```python
from build123d import *
from OCP.BRepFilletAPI import BRepFilletAPI_MakeFillet

# Parameters (mm, degrees)
EXTRUDE_1_DEPTH           = 7.6
SKETCH_3_R                = 1.65
CUT_EXTRUDE_2_DEPTH       = 25.678475018
SKETCH_5_W                = 30
SKETCH_5_H                = 14
EXTRUDE_3_DEPTH           = 3
CUT_EXTRUDE_7_DEPTH       = 0.2
EXTRUDE_9_DEPTH           = 4.5
EXTRUDE_9_DEPTH_BACK      = 1.5
SKETCH_24_R               = 2
CUT_EXTRUDE_8_DEPTH       = 52.317437946
EXTRUDE_10_DEPTH          = 4.5
EXTRUDE_10_DEPTH_BACK     = 1.5
SKETCH_28_R               = 2
CUT_EXTRUDE_9_DEPTH       = 10
FILLET_1_R                = 5
EXTRUDE_11_DEPTH          = 4.5
FILLET_3_R                = 2.2
EXTRUDE_12_DEPTH          = 1.5
SKETCH_33_R               = 4.1
CUT_EXTRUDE_10_DEPTH      = 4.2
CUT_EXTRUDE_START         = -4.2
SKETCH_35_R               = 4.1
CUT_EXTRUDE_11_DEPTH      = 4.2
SKETCH_36_W               = 21
SKETCH_36_H               = 3.5
CUT_EXTRUDE_12_DEPTH      = 30
EXTRUDE_16_DEPTH          = 16
SKETCH_44_R               = 1.6
CUT_EXTRUDE_15_DEPTH      = 6
FILLET_4_R1               = 2
FILLET_4_R2               = 1
FILLET_5_R                = 2
FILLET_4_OF_MIRROR_1_R1   = 2
FILLET_4_OF_MIRROR_1_R2   = 1
FILLET_5_OF_MIRROR_1_R    = 2
MIRROR_START              = -11
MIRROR_2_DEPTH            = 6
MIRROR_2_2_OUTLINE_R      = 1.6
MIRROR_2_2_DEPTH          = 3
SKETCH_45_W               = 21
SKETCH_45_H               = 2
CUT_EXTRUDE_16_DEPTH      = 85.096611109
CUT_EXTRUDE_17_DEPTH      = 87.210440203
CUT_EXTRUDE_17_DEPTH_BACK = 87.210440203
FILLET_6_R                = 0.5


# Read off the part's stored shape, not the designer's step: 镜向2
with BuildPart() as part:
    # 草图1 → 凸台-拉伸1 (new body)
    with BuildSketch(Plane(origin=(0, 0, 0), x_dir=(1, 0, 0), z_dir=(0, 1, 0))):
        with BuildLine():
            Line((0, 5), (15, 5))
            Line((15, 5), (22.940512837, 5))
            Line((22.940512837, 5), (20, 0))
            ThreePointArc((20, 0), (18.535533906, -3.535533906), (15, -5))
            Line((15, -5), (0, -5))
            ThreePointArc((0, -5), (-3.535533906, -3.535533906), (-5, 0))
            Line((-5, 0), (-7.940512837, 5))
            Line((-7.940512837, 5), (0, 5))
        make_face()
    extrude(amount=EXTRUDE_1_DEPTH)

    # 草图3 → 切除-拉伸2 (cut, through all)
    with BuildSketch(Plane(origin=(0, 7.6, 0), x_dir=(1, 0, 0), z_dir=(0, 1, 0))):
        with Locations(Location((0, 0, 0), (0, 0, 270))):
            Circle(SKETCH_3_R)
        with Locations(Location((15, 0, 0), (0, 0, 270))):
            Circle(SKETCH_3_R)
    extrude(amount=-CUT_EXTRUDE_2_DEPTH, mode=Mode.SUBTRACT)

    # 草图5 → 凸台-拉伸3 (add)
    with BuildSketch(Plane(origin=(0, 0, -5), x_dir=(-1, 0, 0), z_dir=(0, 0, -1))):
        with Locations((-7.5, 3.8)):
            Rectangle(SKETCH_5_W, SKETCH_5_H)
    extrude(amount=EXTRUDE_3_DEPTH)

    # 草图10 → 切除-拉伸7 (cut)
    with BuildSketch(Plane.XZ):
        with BuildLine():
            Line((0, 5), (15, 5))
            ThreePointArc((15, 5), (20, 0), (15, -5))
            Line((15, -5), (0, -5))
            ThreePointArc((0, -5), (-5, 0), (0, 5))
        make_face()
    extrude(amount=-CUT_EXTRUDE_7_DEPTH, mode=Mode.SUBTRACT)

    # 草图21 → 凸台-拉伸9 (add, two sides: drawn at the far end of the back side and taken through both)
    with BuildSketch(Plane(origin=(22.5, 0, 0), x_dir=(0, 0, -1), z_dir=(1, 0, 0)).offset(-EXTRUDE_9_DEPTH_BACK)):
        with BuildLine():
            Line((5, 10.8), (29, 10.8))
            ThreePointArc((29, 10.8), (36, 3.8), (29, -3.2))
            Line((29, -3.2), (5, -3.2))
            Line((5, -3.2), (5, 10.8))
        make_face()
    extrude(amount=EXTRUDE_9_DEPTH + EXTRUDE_9_DEPTH_BACK)

    # 草图24 → 切除-拉伸8 (cut, through all)
    with BuildSketch(Plane(origin=(27, 0, 0), x_dir=(0, 0, -1), z_dir=(1, 0, 0))):
        with Locations((28, 4.5)):
            Circle(SKETCH_24_R)
    extrude(amount=-CUT_EXTRUDE_8_DEPTH, mode=Mode.SUBTRACT)

    # 草图25 → 凸台-拉伸10 (add, two sides: drawn at the far end of the back side and taken through both)
    with BuildSketch(Plane.ZY.offset(7.5).offset(-EXTRUDE_10_DEPTH_BACK)):
        with BuildLine():
            Line((-5, -3.2), (-29, -3.2))
            ThreePointArc((-29, -3.2), (-36, 3.8), (-29, 10.8))
            Line((-29, 10.8), (-5, 10.8))
            Line((-5, 10.8), (-5, -3.2))
        make_face()
    extrude(amount=EXTRUDE_10_DEPTH + EXTRUDE_10_DEPTH_BACK)

    # 草图28 → 切除-拉伸9 (cut)
    with BuildSketch(Plane(origin=(-6, 0, 0), x_dir=(0, 0, -1), z_dir=(1, 0, 0))):
        with Locations((28, 4.5)):
            Circle(SKETCH_28_R)
    extrude(amount=-CUT_EXTRUDE_9_DEPTH, mode=Mode.SUBTRACT)

    # 圆角1
    fillet_1_edges = [part.edges().sort_by_distance(p)[0] for p in [
        (-6, 3.8, -8),
        (21, 3.8, -8),
    ]]
    fillet(fillet_1_edges, radius=FILLET_1_R)

    # 草图30 → 凸台-拉伸11 (add)
    with BuildSketch(Plane(origin=(0, 7.6, 0), x_dir=(1, 0, 0), z_dir=(0, 1, 0))):
        Polygon((10, -70), (13.5, -70), (13.5, -75), (1.5, -75), (1.5, -70), (5, -70), (5, 2.116473595), (10, 2.116473595), align=None)
    extrude(amount=EXTRUDE_11_DEPTH)

    # 圆角3
    fillet_3_edges = [part.edges().sort_by_distance(p)[0] for p in [
        (-12, 3.8, -5),
        (-7.940512837, 3.8, -5),
        (22.940512837, 3.8, -5),
        (27, 3.8, -5),
    ]]
    fillet(fillet_3_edges, radius=FILLET_3_R)

    # 草图31 → 凸台-拉伸12 (add)
    with BuildSketch(Plane.XZ.offset(-7.6)):
        Polygon((5, 70), (5, 5), (10, 5), (10, 70), (13.5, 70), (13.5, 75), (1.5, 75), (1.5, 70), align=None)
    extrude(amount=EXTRUDE_12_DEPTH)

    # 草图33 → 切除-拉伸10 (cut)
    with BuildSketch(Plane.ZY.offset(-21)):
        with Locations((-28, 4.5)):
            Circle(SKETCH_33_R)
    extrude(amount=-CUT_EXTRUDE_10_DEPTH, mode=Mode.SUBTRACT)

    # 草图35 → 切除-拉伸11 (cut)
    with BuildSketch(Plane(origin=(-6, 0, 0), x_dir=(0, 0, -1), z_dir=(1, 0, 0)).offset(CUT_EXTRUDE_START)):
        with Locations(Location((28, 4.5, 0), (0, 0, 180))):
            Circle(SKETCH_35_R)
    extrude(amount=CUT_EXTRUDE_11_DEPTH, mode=Mode.SUBTRACT)

    # 草图36 → 切除-拉伸12 (cut)
    with BuildSketch(Plane(origin=(0, 10.8, 0), x_dir=(1, 0, 0), z_dir=(0, 1, 0))):
        with Locations((7.5, 6.75)):
            Rectangle(SKETCH_36_W, SKETCH_36_H)
    extrude(amount=-CUT_EXTRUDE_12_DEPTH, mode=Mode.SUBTRACT)

    # 草图41 → 凸台-拉伸16 (add)
    with BuildSketch(Plane(origin=(0, 10.8, 0), x_dir=(1, 0, 0), z_dir=(0, 1, 0))):
        Polygon((17.5, 11), (11.5, 11), (11.5, 8), (18, 8), (18, 5), (24.8, 5), (24.8, 11), align=None)
    extrude_16 = extrude(amount=EXTRUDE_16_DEPTH)

    # 草图44 → 切除-拉伸15 (cut)
    with BuildSketch(Plane(origin=(0, 0, -11), x_dir=(-1, 0, 0), z_dir=(0, 0, -1))):
        with Locations((-14.5, 23.3)):
            Circle(SKETCH_44_R)
    cut_extrude_15 = extrude(amount=-CUT_EXTRUDE_15_DEPTH, mode=Mode.SUBTRACT)

    # 圆角4: one fillet with a radius per group of edges: ONE call of the kernel's fillet builder (fillet() takes one radius for all edges)
    fillet_4_edges_1 = [part.edges().sort_by_distance(p)[0] for p in [
        (11.5, 10.8, -9.5),
    ]]
    fillet_4_edges_2 = [part.edges().sort_by_distance(p)[0] for p in [
        (11.5, 26.8, -9.5),
    ]]
    fillet_4 = BRepFilletAPI_MakeFillet(part.part.solid().wrapped)
    for e in fillet_4_edges_1:
        fillet_4.Add(FILLET_4_R1, e.wrapped)
    for e in fillet_4_edges_2:
        fillet_4.Add(FILLET_4_R2, e.wrapped)
    add(Compound.cast(fillet_4.Shape()), mode=Mode.REPLACE)

    # 圆角5
    fillet_5_edges = [part.edges().sort_by_distance(p)[0] for p in [
        (24.8, 26.8, -8),
    ]]
    fillet(fillet_5_edges, radius=FILLET_5_R)

    # 镜向1: 凸台-拉伸16, 切除-拉伸15 across plane
    add(extrude_16.mirror(Plane(origin=(7.5, 0, 0), x_dir=(0, 0, 1), z_dir=(1, 0, 0))))
    add(cut_extrude_15.mirror(Plane(origin=(7.5, 0, 0), x_dir=(0, 0, 1), z_dir=(1, 0, 0))), mode=Mode.SUBTRACT)

    # 圆角4 of 镜向1: one fillet with a radius per group of edges: ONE call of the kernel's fillet builder (fillet() takes one radius for all edges)
    fillet_4_of_mirror_1_edges_1 = [part.edges().sort_by_distance(p)[0] for p in [
        (3.5, 10.8, -9.5),
    ]]
    fillet_4_of_mirror_1_edges_2 = [part.edges().sort_by_distance(p)[0] for p in [
        (3.5, 26.8, -9.5),
    ]]
    fillet_4_of_mirror_1 = BRepFilletAPI_MakeFillet(part.part.solid().wrapped)
    for e in fillet_4_of_mirror_1_edges_1:
        fillet_4_of_mirror_1.Add(FILLET_4_OF_MIRROR_1_R1, e.wrapped)
    for e in fillet_4_of_mirror_1_edges_2:
        fillet_4_of_mirror_1.Add(FILLET_4_OF_MIRROR_1_R2, e.wrapped)
    add(Compound.cast(fillet_4_of_mirror_1.Shape()), mode=Mode.REPLACE)

    # 圆角5 of 镜向1
    fillet_5_of_mirror_1_edges = [part.edges().sort_by_distance(p)[0] for p in [
        (-9.8, 26.8, -8),
    ]]
    fillet(fillet_5_of_mirror_1_edges, radius=FILLET_5_OF_MIRROR_1_R)

    # 镜向2 outline → 镜向2 (add)
    with BuildSketch(Plane.XY.offset(MIRROR_START)):
        with BuildLine():
            Line((18, -3.2), (18, -19.2))
            Line((18, -19.2), (22.8, -19.2))
            ThreePointArc((22.8, -19.2), (24.214213562, -18.614213562), (24.8, -17.2))
            Line((24.8, -17.2), (24.8, -3.2))
            Line((24.8, -3.2), (18, -3.2))
        make_face()
        with BuildLine():
            Line((-3, -19.2), (-3, -3.2))
            Line((-3, -3.2), (-9.8, -3.2))
            Line((-9.8, -3.2), (-9.8, -17.2))
            ThreePointArc((-9.8, -17.2), (-9.214213562, -18.614213562), (-7.8, -19.2))
            Line((-7.8, -19.2), (-3, -19.2))
        make_face()
    extrude(amount=MIRROR_2_DEPTH)

    # Mirror 2 2 outline → Mirror 2 2 (add)
    # profile 1 of 2: a face of its own
    with BuildSketch(Plane.XY.offset(MIRROR_START)):
        with BuildLine():
            Line((12.5, -19.2), (18, -19.2))
            Line((18, -19.2), (18, -3.2))
            Line((18, -3.2), (13.5, -3.2))
            ThreePointArc((13.5, -3.2), (12.085786438, -3.785786438), (11.5, -5.2))
            Line((11.5, -5.2), (11.5, -18.2))
            ThreePointArc((11.5, -18.2), (11.792893219, -18.907106781), (12.5, -19.2))
        make_face()
        with Locations((14.5, -15.7)):
            Circle(MIRROR_2_2_OUTLINE_R, mode=Mode.SUBTRACT)
    # profile 2 of 2: a face of its own
    with BuildSketch(Plane.XY.offset(MIRROR_START)):
        with BuildLine():
            Line((1.5, -3.2), (-3, -3.2))
            Line((-3, -3.2), (-3, -19.2))
            Line((-3, -19.2), (2.5, -19.2))
            ThreePointArc((2.5, -19.2), (3.207106781, -18.907106781), (3.5, -18.2))
            Line((3.5, -18.2), (3.5, -5.2))
            ThreePointArc((3.5, -5.2), (2.914213562, -3.785786438), (1.5, -3.2))
        make_face()
        with Locations((0.5, -15.7)):
            Circle(MIRROR_2_2_OUTLINE_R, mode=Mode.SUBTRACT)
    extrude(amount=MIRROR_2_2_DEPTH)

    # 草图45 → 切除-拉伸16 (cut, through all)
    with BuildSketch(Plane(origin=(0, 7.6, 0), x_dir=(1, 0, 0), z_dir=(0, 1, 0))):
        with Locations((7.5, 4)):
            Rectangle(SKETCH_45_W, SKETCH_45_H)
    extrude(amount=-CUT_EXTRUDE_16_DEPTH, mode=Mode.SUBTRACT)

    # 草图46 → 切除-拉伸17 (cut, two sides: drawn at the far end of the back side and taken through both)
    with BuildSketch(Plane.ZY.offset(-21).offset(-CUT_EXTRUDE_17_DEPTH_BACK)):
        with BuildLine():
            ThreePointArc((-29, 10.8), (-33.807417596, 3.8), (-29, -3.2))
            ThreePointArc((-29, -3.2), (-36, 3.8), (-29, 10.8))
        make_face()
    extrude(amount=CUT_EXTRUDE_17_DEPTH + CUT_EXTRUDE_17_DEPTH_BACK, mode=Mode.SUBTRACT)

    # 圆角6
    fillet_6_edges = [part.edges().sort_by_distance(p)[0] for p in [
        (21, 3.8, -33.807417596),
        (-6, 3.8, -33.807417596),
    ]]
    fillet(fillet_6_edges, radius=FILLET_6_R - 0.0001)  # a hair under: the kernel refuses the full size


solid = part.part
```
Can you work these out from the model? Positions are in its coordinate system, mm. A direction names the side the tool comes from. Coordinates: 2 decimals unless noted, no trailing zeros. Loops run counter-clockwise (first coordinate to the right, second up) from the corner with the lowest first, then second, coordinate; pieces in that order, holes last. Notation, with made-up numbers: (-26, 69) -> (-2, 69) arc R25 ccw to (-2, 94) -> close; hole circle Ø4 at (18, 62). An arc over 180 degrees is marked (long way). Put each result on its own line as item: value. Start each with the question number.
Q1. I want a section at B-B (y = -15.7). Write out the boundary of the cut face in (x, z).
Q2. I want a section at A-A (y = -7). Write out the boundary of the cut face in (x, z), plus the area to 3 significant figures.
Q3. For faces 4 (the face through (-5, 4, -10)), 5 (the face through (2.93, -3.8, -9.52)), 6 (the face through (3.5, -12, -10)), which set-ups out of +Z, -Z, +X, -X, +Y, -Y let a thin tool reach every point of the face, with its end or its side?
Q4. Thinking about a two-plate mould opening in X: for faces 1 (the face through (16.1, 23.37, -9.52)), 2 (the face through (8, 12.1, 44)), 3 (the face through (-9.8, 18, -8)), which applies, pulls with the +X half, pulls with the -X half, needs draft (parallel to the pull), parting line crosses it, or undercut?
Q5. I want a section at C-C (z = -10). Count the separate pieces of the cut face and the enclosed holes in it, plus the area to 3 significant figures.
Q6. If I drill on line 1 (X direction, y = 5, z = 0); line 2 (Y direction, x = 14.5, z = -9.3); line 3 (Y direction, x = 0, z = -10), over which ranges is the centre line in solid material (lowest first)? Write a range as [from, to].
Q7. I'm going to push flat-ended pins straight in: P1, Ø14.5, axis at x = -2.5, y = -8, coming from the -Z side; P2, Ø1, axis at x = 7, z = 39.5, coming from the -Y side; P3, Ø8, axis at x = 3.5, y = 18.5, coming from the +Z side. Where does each tip first touch, or does it pass through?
Q8. I want a section at D-D (z = 36.5). Write out the boundary of the cut face in (x, y).
Taken from the geometry:
1. outline: (-9.8, -11) -> (-1.1, -11) -> (-1.1, -8) -> (-3, -8) -> (-3, -5) -> (-9.8, -5) -> close; (2.1, -11) -> (3.5, -11) -> (3.5, -8) -> (2.1, -8) -> close; (11.5, -11) -> (12.9, -11) -> (12.9, -8) -> (11.5, -8) -> close; (16.1, -11) -> (24.8, -11) -> (24.8, -5) -> (18, -5) -> (18, -8) -> (16.1, -8) -> close
2. outline: (-9.8, -11) -> (3.5, -11) -> (3.5, -8) -> (-3, -8) -> (-3, -5) -> (-9.8, -5) -> close; (11.5, -11) -> (24.8, -11) -> (24.8, -5) -> (18, -5) -> (18, -8) -> (11.5, -8) -> close
2. area: 121 mm2
3. face 4: -Z
3. face 5: +Z, -Z
3. face 6: +Z, -Z, +Y, -Y
4. face 1: undercut
4. face 2: needs draft
4. face 3: pulls with the -X half
5. separate pieces: 2
5. enclosed holes: 4
5. area: 1,010 mm2
6. line 1: x = [-5, -1.65], [1.65, 13.35], [16.65, 20]
6. line 2: y = [-19.2, -17.3], [-14.1, -3.2], [10.8, 21.7], [24.9, 26.8]
6. line 3: y = [-19.2, -17.22], [-14.18, -3.2], [10.8, 21.78], [24.82, 26.8]
7. P1: stops at z = -31.2
7. P2: stops at y = 6.1
7. P3: stops at z = -8
8. outline: (5, 6.1) -> (10, 6.1) -> (10, 12.1) -> (5, 12.1) -> close
